from build123d import *

# Parameters (mm, degrees)
SKETCH1_R           = 2.3
BOSS_EXTRUDE1_DEPTH = 3


with BuildPart() as part:
    # Sketch1 → Boss-Extrude1 (new body)
    with BuildSketch(Plane(origin=(0, 0, 0), x_dir=(0, 0, -1), z_dir=(1, 0, 0))):
        with BuildLine():
            Line((-5.5, 0), (5.5, 0))
            ThreePointArc((5.5, 0), (7.621320344, 0.878679656), (8.5, 3))
            Line((8.5, 3), (8.5, 87))
            ThreePointArc((8.5, 87), (7.621320344, 89.121320344), (5.5, 90))
            Line((5.5, 90), (-5.5, 90))
            ThreePointArc((-5.5, 90), (-7.621320344, 89.121320344), (-8.5, 87))
            Line((-8.5, 87), (-8.5, 3))
            ThreePointArc((-8.5, 3), (-7.621320344, 0.878679656), (-5.5, 0))
        make_face()
        with Locations((0, 10)):
            Circle(SKETCH1_R, mode=Mode.SUBTRACT)
        with Locations(Location((0, 80, 0), (0, 0, 180))):
            Circle(SKETCH1_R, mode=Mode.SUBTRACT)
    extrude(amount=BOSS_EXTRUDE1_DEPTH)


solid = part.part
Can you work these out from the model? Positions are in its coordinate system, mm. Give positions to 0.01 mm unless a question says otherwise; leave off trailing zeros. Loops run counter-clockwise (first coordinate to the right, second up) from the corner with the lowest first, then second, coordinate; pieces in that order, holes last. Notation, with made-up numbers: (55, -32) -> (96, -32) arc R21 ccw to (96, -11) -> close; hole circle Ø4 at (-9, 9.25). An arc over 180 degrees is marked (long way). Write item = value, one per line.
1) I need wall thicknesses on L1, parallel to Y at x = 1.5, z = 0; L2, parallel to Y at x = 1.8, z = 0.75; L3, parallel to Z at x = 1.5, y = 79. Which ranges of each line are inside material? Lowest first, please. Write a range as from..to.
Check result:
L1 = 0..7.7, 12.3..77.7, 82.3..90
L2 = 0..7.83, 12.17..77.83, 82.17..90
L3 = -8.5..-2.07, 2.07..8.5
2) Thinking about a two-plate mould opening in Y: for faces 1 (the cylindrical face through (1.48, 12.28, 0.3)), 2 (the flat face through (1, 46, 8.5)), 3 (the cylindrical face through (1.48, 0.86, -7.6)), which applies, released by +Y, released by -Y, zero draft, split by the parting line, or undercut?
Check result:
face_1 = undercut
face_2 = zero draft
face_3 = released by -Y
3) Suppose I cut it at B-B on x = 1.1. Write out the boundary of the cut face in (y, z).
Check result:
outline = (0, -5.5) arc R3 ccw to (3, -8.5) -> (87, -8.5) arc R3 ccw to (90, -5.5) -> (90, 5.5) arc R3 ccw to (87, 8.5) -> (3, 8.5) arc R3 ccw to (0, 5.5) -> close; hole circle Ø4.6 at (10, 0); hole circle Ø4.6 at (80, 0)
4) Suppose I cut it at A-A on z = 0. Write out the boundary of the cut face in (x, y).
Check result:
outline = (0, 0) -> (3, 0) -> (3, 7.7) -> (0, 7.7) -> close; (0, 12.3) -> (3, 12.3) -> (3, 77.7) -> (0, 77.7) -> close; (0, 82.3) -> (3, 82.3) -> (3, 90) -> (0, 90) -> close
5) Suppose I cut it at C-C on y = 10. Write out the boundary of the cut face in (x, z).
Check result:
outline = (0, -8.5) -> (3, -8.5) -> (3, -2.3) -> (0, -2.3) -> close; (0, 2.3) -> (3, 2.3) -> (3, 8.5) -> (0, 8.5) -> close
